Model file for the job. Use its own axes, mm. Face numbers are marked on the shaded views. A direction names the side the tool comes from. Coordinates: 2 decimals unless noted, no trailing zeros. Order: outer loops, then holes, each group sorted by start corner. A loop starts at its lowest first (then second) coordinate and runs counter-clockwise, first axis right, second up. Notation, with made-up numbers: (72.5, 80) -> (78.5, 80) arc R14 cw to (78.5, 92) -> close; hole circle Ø7 at (52.5, 39.5). An arc over 180 degrees is marked (long way). Use CSV: the item, a comma, the result in double quotes. Start each with the question number.
(1) Probe L1, parallel to Y at x = -5.5, z = -4.5; L2, parallel to X at y = -9, z = -25; L3, parallel to X at y = -3.5, z = 10.5. List the from-to ranges inside material, lowest first.
(2) Pull direction Y, two halves, no side cores. Call the marked faces 3, 4 and 5: pulls with the +Y half, pulls with the -Y half, needs draft (parallel to the pull), parting line crosses it, or undercut.
(3) Cut at B-B on y = -38. Write the cut outline in (x, z).
(4) Cut at C-C on z = -2. Write the cut outline in (x, y).
(5) Cut at A-A on x = 5. Write the cut outline in (y, z).
(6) Tool access for the marked faces 1 and 2: list every direction of +Z, -Z, +X, -X, +Y, -Y with a clear straight run to the whole face (end or side of a thin tool).
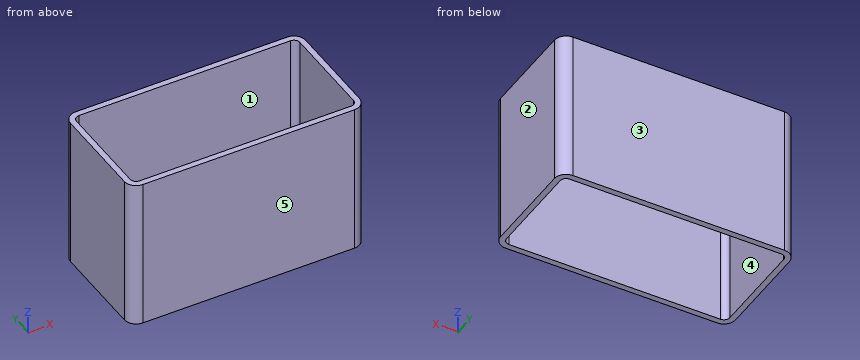
```python
from build123d import *

# Parameters (mm, degrees)
F0_W     = 100
F0_H     = 65
F1_DEPTH = 50
F2_R     = 5
F3_T     = -2.5


with BuildPart() as f1:
    # F0 (on Front) → F1 (new body)
    with BuildSketch(Plane.XZ):
        Rectangle(F0_W, F0_H)
    extrude(amount=F1_DEPTH)

    # F2
    f2_edges = [f1.edges().sort_by_distance(p)[0] for p in [
        (-50, -50, 0),
        (50, -50, 0),
        (-50, 0, 0),
        (50, 0, 0),
    ]]
    fillet(f2_edges, radius=F2_R)

    # F3
    f3_openings = [f1.faces().sort_by_distance(p)[0] for p in [
        (0, -25, 32.5),
        (0, -25, -32.5),
    ]]
    offset(amount=F3_T, openings=f3_openings)


solid = f1.part
```
Outcome:
1,L1,"-50 to -47.5, -2.5 to 0"
1,L2,"-50 to -47.5, 47.5 to 50"
1,L3,"-49.77 to -47, 47 to 49.77"
2,face 3,"pulls with the +Y half"
2,face 4,"undercut"
2,face 5,"pulls with the -Y half"
3,outline,"(-50, -32.5) -> (-47.5, -32.5) -> (-47.5, 32.5) -> (-50, 32.5) -> close; (47.5, -32.5) -> (50, -32.5) -> (50, 32.5) -> (47.5, 32.5) -> close"
4,outline,"(-50, -45) arc R5 ccw to (-45, -50) -> (45, -50) arc R5 ccw to (50, -45) -> (50, -5) arc R5 ccw to (45, 0) -> (-45, 0) arc R5 ccw to (-50, -5) -> close; hole (-47.5, -45) arc R2.5 ccw to (-45, -47.5) -> (45, -47.5) arc R2.5 ccw to (47.5, -45) -> (47.5, -5) arc R2.5 ccw to (45, -2.5) -> (-45, -2.5) arc R2.5 ccw to (-47.5, -5) -> close"
5,outline,"(-50, -32.5) -> (-47.5, -32.5) -> (-47.5, 32.5) -> (-50, 32.5) -> close; (-2.5, -32.5) -> (0, -32.5) -> (0, 32.5) -> (-2.5, 32.5) -> close"
6,face 1,"+Z, -Z"
6,face 2,"+Z, -Z, +X, +Y, -Y"
